from build123d import *

# Parameters (mm, degrees)
SKETCH_1_W                   = 30.5
SKETCH_1_H                   = 30
EXTRUDE_1_DEPTH              = 6
HOLE_WIZARD_M6_1_D           = 6.5
HOLE_WIZARD_M6_1_CSINK_D     = 10
HOLE_WIZARD_M6_1_CSINK_ANGLE = 90
EXTRUDE_3_DEPTH              = 30


with BuildPart() as part:
    # 草图1 → 凸台-拉伸1 (new body)
    with BuildSketch(Plane.XY):
        with Locations((15.25, -15)):
            Rectangle(SKETCH_1_W, SKETCH_1_H)
    extrude(amount=EXTRUDE_1_DEPTH)

    # M6 内六角花形半沉头螺钉的锥形沉头孔1 (through all)
    with Locations(Plane.XY.offset(6)):
        with Locations((8.75, -15), (21.75, -15)):
            CounterSinkHole(HOLE_WIZARD_M6_1_D / 2, HOLE_WIZARD_M6_1_CSINK_D / 2, counter_sink_angle=HOLE_WIZARD_M6_1_CSINK_ANGLE)

    # 草图5 → 凸台-拉伸3 (add)
    with BuildSketch(Plane.XZ.offset(30)):
        with BuildLine():
            ThreePointArc((0.151530772, 7.5), (-12.597922496, 12.856607172), (-7.5, 0.001530928))
            Line((-7.5, 0.001530928), (-7.5, 6))
            Line((-7.5, 6), (0, 6))
            ThreePointArc((0, 6), (0.113551919, 6.746182785), (0.151530772, 7.5))
        make_face()
        with BuildLine():
            ThreePointArc((-7.5, 0.001530928), (-7.424238481, 0.000382742), (-7.348469228, 0))
            ThreePointArc((-7.348469228, 0), (-2.605052738, 1.690524981), (0, 6))
            Line((0, 6), (-7.5, 6))
            Line((-7.5, 6), (-7.5, 0.001530928))
        make_face()
        with BuildLine():
            Line((-7.348469228, 0), (0, 0))
            Line((0, 0), (0, 6))
            ThreePointArc((0, 6), (-2.605052738, 1.690524981), (-7.348469228, 0))
        make_face()
    extrude(amount=-EXTRUDE_3_DEPTH)


solid = part.part
Input: part model. Units: mm. Frame: model coordinates. Round coordinates to 2 decimals unless told otherwise and drop trailing zeros. Order: outer loops, then holes, each group sorted by start corner. A loop starts at its lowest first (then second) coordinate and runs counter-clockwise, first axis right, second up. Notation, with made-up numbers: (60.25, -5) - (85.25, -5) arc R5 ccw to (85.25, 3) - close; hole circle Ø11 at (87, 0). An arc over 180 degrees is marked (long way). Answer as a JSON object with one key per item and string values. Group by question number.
(1) Cut plane D-D (y = -2.75). Return loops of the section in (x, z), then the cut area to 3 significant figures.
(2) Pin query (flat end, axial travel): P1, Ø1, axis at y = -11, z = 9.5, coming from the +X side; P2, Ø9, axis at x = 18.5, y = -7.5, coming from the +Z side; P3, Ø5, axis at x = 8, y = -18, coming from the -Z side; P4, Ø3, axis at x = -1.5, y = -9, coming from the +Z side. Return the tip coordinate at first contact, or that it passes through.
(3) Cut plane A-A (y = -15). Return loops of the section in (x, z), then the cut area to 3 significant figures.
(4) Cut plane B-B (x = 21.75). Return loops of the section in (y, z), then the cut area to 3 significant figures.
(5) Draft query along Y for faces 1 (the face through (9.173, -11.778, 2.095)), 2 (the face through (2, 0, 4)), 3 (the face through (30.5, -15, 3)). Return one class per face: released by +Y, released by -Y, zero draft, split by the parting line, or undercut.
(6) Cut plane C-C (z = 1.25). Return loops of the section in (x, y).
(7) Material intervals for probe 1 along X at (y, z) = (-15, 1.7); probe 2 along Y at (x, z) = (8.75, 2.2); probe 3 along X at (y, z) = (-15, 0.95), sorted ascending. Write a range as from..to.
Here are the results:
{
 "1": {"outline": "(-7.5, 0) arc R7.5 ccw to (-7.35, 0) - (30.5, 0) - (30.5, 6) - (0, 6) arc R7.5 ccw (long way) to start", "area": "371 mm^2"},
 "2": {"P1": "stops at x = 0", "P2": "stops at z = 6", "P3": "stops at z = 0", "P4": "stops at z = 13.61"},
 "3": {"outline": "(-7.5, 0) arc R7.5 ccw to (-7.35, 0) - (5.5, 0) - (5.5, 4.25) - (3.75, 6) - (0, 6) arc R7.5 ccw (long way) to start; (12, 0) - (18.5, 0) - (18.5, 4.25) - (16.75, 6) - (13.75, 6) - (12, 4.25) - close; (25, 0) - (30.5, 0) - (30.5, 6) - (26.75, 6) - (25, 4.25) - close", "area": "287 mm^2"},
 "4": {"outline": "(-30, 0) - (-18.25, 0) - (-18.25, 4.25) - (-20, 6) - (-30, 6) - close; (-11.75, 0) - (0, 0) - (0, 6) - (-10, 6) - (-11.75, 4.25) - close", "area": "138 mm^2"},
 "5": {"face 1": "undercut", "face 2": "released by +Y", "face 3": "zero draft"},
 "6": {"outline": "(-11.49, -30) - (30.5, -30) - (30.5, 0) - (-11.49, 0) - close; hole circle Ø6.5 at (8.75, -15); hole circle Ø6.5 at (21.75, -15)"},
 "7": {"probe 1": "x = -12.1..5.5, 12..18.5, 25..30.5", "probe 2": "y = -30..-18.25, -11.75..0", "probe 3": "x = -11..5.5, 12..18.5, 25..30.5"}
}
